```python
from build123d import *

# Parameters (mm, degrees)
CROQUIS1_R              = 2.5
SALIENTE_EXTRUIR1_DEPTH = 1.5
MATRIZL1_COUNT          = 2
MATRIZL1_PITCH          = 30.5
MATRIZL1_COUNT_DIR2     = 2
MATRIZL1_PITCH_DIR2     = 30.5


with BuildPart() as part:
    # Croquis1 → Saliente-Extruir1 (new body)
    with BuildSketch(Plane.XY):
        with BuildLine():
            Line((17.88322612, 13.695977011), (17.88322612, -17.304022989))
            ThreePointArc((17.88322612, -17.304022989), (13.88322612, -21.304022989), (9.88322612, -17.304022989))
            Line((9.88322612, -17.304022989), (-11.66677388, -17.304022989))
            ThreePointArc((-11.66677388, -17.304022989), (-15.66677388, -21.304022989), (-19.66677388, -17.304022989))
            Line((-19.66677388, -17.304022989), (-19.66677388, 13.695977011))
            ThreePointArc((-19.66677388, 13.695977011), (-15.66677388, 17.695977011), (-11.66677388, 13.695977011))
            Line((-11.66677388, 13.695977011), (9.88322612, 13.695977011))
            ThreePointArc((9.88322612, 13.695977011), (13.88322612, 17.695977011), (17.88322612, 13.695977011))
        make_face()
        with Locations((-16.14177388, 13.445977011)):
            Circle(CROQUIS1_R, mode=Mode.SUBTRACT)
        with Locations((14.35822612, 13.445977011)):
            Circle(CROQUIS1_R, mode=Mode.SUBTRACT)
        with Locations((14.35822612, -17.054022989)):
            Circle(CROQUIS1_R, mode=Mode.SUBTRACT)
        with Locations((-16.14177388, -17.054022989)):
            Circle(CROQUIS1_R, mode=Mode.SUBTRACT)
    extrude(amount=SALIENTE_EXTRUIR1_DEPTH)

    # Croquis3 → Revolución1 (revolve)
    with BuildSketch(Plane(origin=(0, -17.054022989, 0), x_dir=(-1, 0, 0), z_dir=(0, -1, 0)), mode=Mode.PRIVATE) as revoluci_n1_sk:
        Polygon((18.64177388, -1.5), (19.64177388, -1.5), (19.64177388, -2.5), (17.64177388, -2.5), (17.64177388, 5), (19.64177388, 5), (19.64177388, 0), (18.64177388, 0), align=None)
    revoluci_n1 = revolve(revoluci_n1_sk.sketch.rotate(Axis((-16.14177388, -17.054022989, 2.5), (0, 0, -1)), 180), axis=Axis((-16.14177388, -17.054022989, 2.5), (0, 0, -1)))

    # MatrizL1: Revoluci_n1 2 × 2
    with Locations(*[(i * MATRIZL1_PITCH, j * MATRIZL1_PITCH_DIR2, 0) for i in range(MATRIZL1_COUNT) for j in range(MATRIZL1_COUNT_DIR2) if (i, j) != (0, 0)]):
        add(revoluci_n1)


solid = part.part
```
CAD build for the part. Positions are in the model's coordinates, mm. A direction names the side the tool comes from. Round coordinates to 2 decimals unless told otherwise and drop trailing zeros. Loops run counter-clockwise (first coordinate to the right, second up) from the corner with the lowest first, then second, coordinate; pieces in that order, holes last. Notation, with made-up numbers: M 54.25,29.25 L 62.25,29.25 A22 ccw 62.25,60.25 Z; hole C 22,57.25 d1. An arc over 180 degrees is marked long. Return JSON: item names as keys, results as strings. Group by question number.
(1) Saw through at C-C, the plane y = 14.5. Give the number of separate pieces and of enclosed holes in the cut face, and give its area (3 significant figures).
(2) Mould opens along Y. For faces 1 (the cylindrical face through (-12.8, 12.4, 2)), 2 (the cylindrical face through (13.971, -21.303, 0.74)), 3 (the cylindrical face through (13.903, 9.976, -2.465)), 4 (the flat face through (-19.667, -2, 1)) say: +Y half, -Y half, draft (parallel to the pull), parting line (faces both ways), or undercut.
(3) Saw through at B-B, the plane y = -19. List the corners of the cut face in (x, z).
(4) Saw through at D-D, the plane x = -2. List the corners of the cut face in (y, z), and give its area (3 significant figures).
(5) Wall check: probe 1 along X at (y, z) = (-19, -2); probe 2 along Z at (x, y) = (16.5, 9.5); probe 3 along Y at (x, z) = (11.5, 2.25). Give the ranges that are in metal, low to high. Write a range as [from, to].
(6) Drop flat-ended pins along their axis: P1, Ø19, axis at x = -4.5, y = -10.5, coming from the -Z side; P2, Ø1.2, axis at x = 4, z = 1, coming from the +Y side; P3, Ø8, axis at x = -0.5, y = 8, coming from the +Z side. Give the stop position or say it passes through.
(7) Saw through at A-A, the plane z = -0.75. List the corners of the cut face in (x, y).
(8) Tool access for faces 5 (the cylindrical face through (-12.91, -15.71, 2.01)), 6 (the cylindrical face through (-12.91, -15.71, -2.46)), 7 (the flat face through (-1, 13.696, 1)), 8 (the flat face through (-18, -17, -5)), 9 (the cylindrical face through (-17.247, 12.432, -1.303)): list every direction of +Z, -Z, +X, -X, +Y, -Y with a clear straight run to the whole face (end or side of a thin tool).
Answer list:
{
 "1": {"separate pieces": "4", "enclosed holes": "0", "area": "71.6 mm2"},
 "2": {"face 1": "undercut", "face 2": "-Y half", "face 3": "undercut", "face 4": "draft"},
 "3": {"outline": "M -19.29,0 L -19.05,0 L -19.05,-5 L -13.23,-5 L -13.23,0 L -12.04,0 L -12.04,1.5 L -13.23,1.5 L -13.23,2.5 L -19.05,2.5 L -19.05,1.5 L -19.29,1.5 Z; M 10.26,0 L 11.45,0 L 11.45,-5 L 17.27,-5 L 17.27,0 L 17.51,0 L 17.51,1.5 L 17.27,1.5 L 17.27,2.5 L 11.45,2.5 L 11.45,1.5 L 10.26,1.5 Z"},
 "4": {"outline": "M -17.3,0 L 13.7,0 L 13.7,1.5 L -17.3,1.5 Z", "area": "46.5 mm2"},
 "5": {"probe 1": "[-19.05, -13.23], [11.45, 17.27]", "probe 2": "[0, 1.5]", "probe 3": "[-19.07, -15.03], [11.43, 15.47]"},
 "6": {"P1": "z = 0", "P2": "y = 13.7", "P3": "z = 1.5"},
 "7": {"outline": "C -16.14,-17.05 d7; C -16.14,13.45 d7; C 14.36,-17.05 d7; C 14.36,13.45 d7; hole C -16.14,-17.05 d3; hole C -16.14,13.45 d3; hole C 14.36,-17.05 d3; hole C 14.36,13.45 d3"},
 "8": {"face 5": "+Z", "face 6": "-Z", "face 7": "+Z, -Z, +Y", "face 8": "-Z, +X, -X, +Y, -Y", "face 9": "+Z, -Z"}
}
